The model under review builds one solid part; all positions refer to its coordinate system, in mm. Round coordinates to 2 decimals unless told otherwise and drop trailing zeros. Write each loop counter-clockwise with the first axis right and the second up, starting at its lowest first coordinate (ties: lowest second). Pieces come first, ordered by that corner, then holes. Notation, with made-up numbers: (4.5, 37.5) - (42.5, 37.5) arc R13 cw to (42.5, 62.5) - close; hole circle Ø1 at (-40, 57.25). An arc over 180 degrees is marked (long way). Use one line per item in the form item = value.
Autodesk Inventor part; units mm, degrees
ref_plane "YZ Plane" through (0, 0, 0) normal (1, 0, 0) x (0, 1, 0)
ref_plane "XZ Plane" through (0, 0, 0) normal (0, 1, 0) x (-1, 0, 0)
ref_plane "XY Plane" through (0, 0, 0) normal (0, 0, 1) x (1, 0, 0)
sketch "Sketch1" plane through (0, 0, 0) normal (0, 0, 1) x (1, 0, 0)
  circle A0 centre (0, 0) radius 6
  dimension "d0" = 12
extrude "Extrusion1" add sketch "Sketch1" along normal blind 326
sketch "Sketch2" plane through (0, 0, 326) normal (0, 0, 1) x (1, 0, 0)
  circle A0 centre (0, 0) radius 4
  dimension "d3" = 8
extrude "Extrusion2" add sketch "Sketch2" along normal blind 12
thread "Thread1"
sketch "Sketch3" plane through (0, 0, 0) normal (0, 0, -1) x (-1, 0, 0)
  circle A0 centre (0, 0) radius 5
  circle A1 centre (0, 0) radius 6
  dimension "d8" = 10
  dimension "d9" = 12
extrude "Extrusion3" cut sketch "Sketch3" against normal blind 14
properties part number "Tornillo de Vínculo Cabezal" material "Steel"
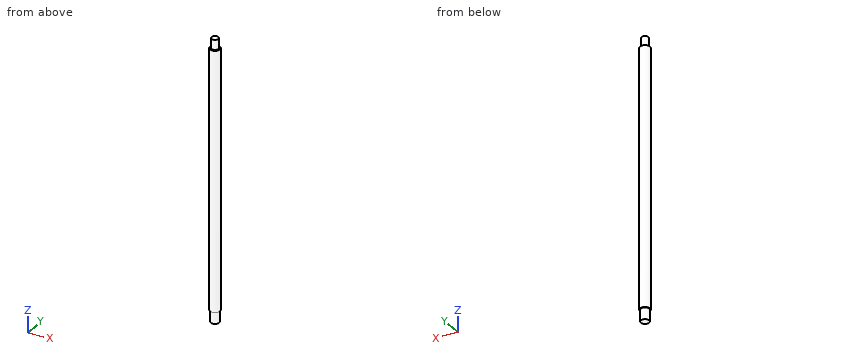
(1) Add section A-A on y = 0. Write out the cut boundary in (x, z).
Geometry results:
outline = (-6, 14) - (-5, 14) - (-5, 0) - (5, 0) - (5, 14) - (6, 14) - (6, 326) - (4, 326) - (4, 338) - (-4, 338) - (-4, 326) - (-6, 326) - close
(2) Add section C-C on z = 88. Write out the cut boundary in (x, y).
Geometry results:
outline = circle Ø12 at (0, 0)
(3) Insertion check: P1, Ø2, axis at y = -4, z = 265, coming from the +X side; P2, Ø3, axis at y = 3, z = 120, coming from the -X side. Each pin has a flat end and moves straight along its axis. Give the tip position at first contact, or say it passes through.
Geometry results:
P1 = 5.2
P2 = -5.81
(4) To check wall thickness, follow L1, parallel to Y at x = -4.5, z = 21.5; L2, parallel to Y at x = 3.25, z = 213; L3, parallel to Z at x = 1.25, y = -5.25. State the ranges of each line that lie inside material, in increasing order.
Geometry results:
L1 = -3.97 to 3.97
L2 = -5.04 to 5.04
L3 = 14 to 326
